from build123d import *

# Parameters (mm, degrees)
BOSS_EXTRUDE1_DEPTH    = 19.05
CONVERT_SOLID1_START   = -19.05
CONVERT_SOLID1_DEPTH   = 38.1
CONVERT_SOLID1_2_DEPTH = 38.1
SKETCH2_W              = 1.8542
SKETCH2_H              = 5.2324
CUT_EXTRUDE1_DEPTH     = 3.175


# Read off the part's stored shape, not the designer's step: SharpBend1
with BuildPart() as part:
    # Sketch1 → Boss-Extrude1 (new, symmetric)
    with BuildSketch(Plane(origin=(0, 0, 0), x_dir=(1, 0, 0), z_dir=(0, 0, -1))):
        Polygon((1.6002, -2.6162), (-6.35, -2.6162), (-6.35, -1.016), (0, -1.016), (0, 1.016), (-6.35, 1.016), (-6.35, 2.6162), (1.6002, 2.6162), align=None)
    extrude(amount=BOSS_EXTRUDE1_DEPTH, both=True)

    # Convert-Solid1 outline → Convert-Solid1 (cut)
    with BuildSketch(Plane.XY.offset(CONVERT_SOLID1_START)):
        with BuildLine():
            Line((1.6002, -2.6162), (1.6002, -0.9906))
            ThreePointArc((1.6002, -0.9906), (1.124072783, -2.140072783), (-0.0254, -2.6162))
            Line((-0.0254, -2.6162), (1.6002, -2.6162))
        make_face()
        with BuildLine():
            ThreePointArc((-0.0254, 2.6162), (1.124072783, 2.140072783), (1.6002, 0.9906))
            Line((1.6002, 0.9906), (1.6002, 2.6162))
            Line((1.6002, 2.6162), (-0.0254, 2.6162))
        make_face()
    extrude(amount=CONVERT_SOLID1_DEPTH, mode=Mode.SUBTRACT)

    # Convert-Solid1 2 outline → Convert-Solid1 2 (add)
    with BuildSketch(Plane.XY.offset(CONVERT_SOLID1_START)):
        with BuildLine():
            Line((0, -1.016), (0, -0.9906))
            ThreePointArc((0, -0.9906), (-0.007439488, -1.008560512), (-0.0254, -1.016))
            Line((-0.0254, -1.016), (0, -1.016))
        make_face()
        with BuildLine():
            ThreePointArc((-0.0254, 1.016), (-0.007439488, 1.008560512), (0, 0.9906))
            Line((0, 0.9906), (0, 1.016))
            Line((0, 1.016), (-0.0254, 1.016))
        make_face()
    extrude(amount=CONVERT_SOLID1_2_DEPTH)

    # Sketch2 → Cut-Extrude1 (cut, symmetric)
    with BuildSketch(Plane.XY):
        with Locations((0.6731, 0)):
            Rectangle(SKETCH2_W, SKETCH2_H)
    extrude(amount=CUT_EXTRUDE1_DEPTH, both=True, mode=Mode.SUBTRACT)


solid = part.part
Here's how the part is built. I have some questions about the finished solid (model axes, mm). A direction names the side the tool comes from. Coordinates: 2 decimals unless noted, no trailing zeros. Order: outer loops, then holes, each group sorted by start corner. A loop starts at its lowest first (then second) coordinate and runs counter-clockwise, first axis right, second up. Notation, with made-up numbers: (-10, 37) - (17, 37) arc R19 cw to (17, 68) - close; hole circle Ø4 at (27, 52.5). An arc over 180 degrees is marked (long way). Use CSV: the item, a comma, the result in double quotes. Start each with the question number.
1. Suppose I cut it at D-D on y = -2.2. List the corners of the cut face in (x, z) for me (3 decimals), then the cut area to 3 significant figures.
2. Suppose I cut it at A-A on y = 0.05. List the corners of the cut face in (x, z) for me (3 decimals), then the cut area to 3 significant figures.
3. Suppose I cut it at B-B on x = -0.75. List the corners of the cut face in (y, z) for me.
4. Please list where these lines run through material, in increasing order: line 1 (Z direction, x = 1.25, y = -0.95) (3 decimals); line 2 (Y direction, x = -3.5, z = -15); line 3 (X direction, y = -1.15, z = 7.5). Write a range as from..to.
5. I'm going to push flat-ended pins straight in: pin 1 (1.6 mm diameter, centred on y = 0, z = 9, fed in from -X); pin 2 (1.3 mm diameter, centred on y = 2, z = -0.5, fed in from +X); pin 3 (2 mm diameter, centred on x = 0.5, z = 8.5, fed in from -Y). Where does each tip first touch, or does it pass through?
6. For faces 5 (the face through (-3, 1.016, 0)), 6 (the face through (-6.35, -2, 0)), 7 (the face through (-0.254, -2, 0)), which set-ups out of +Z, -Z, +X, -X, +Y, -Y let a thin tool reach every point of the face, with its end or its side?
7. If we mould it in two halves opening along Z, with no side actions, what happens to faces 1 (the face through (0, 0, -11)), 2 (the face through (-2.4, 1.2, 19.05)), 3 (the face through (1, 0, 3.175)), 4 (the face through (1, 0, -3.175))? For each: +Z half, -Z half, draft (parallel to the pull), parting line (faces both ways), or undercut.
Output:
1,outline,"(-6.35, -19.05) - (1.061, -19.05) - (1.061, -3.175) - (-0.254, -3.175) - (-0.254, 3.175) - (1.061, 3.175) - (1.061, 19.05) - (-6.35, 19.05) - close"
1,area,"274 mm2"
2,outline,"(0, -19.05) - (1.6, -19.05) - (1.6, -3.175) - (0, -3.175) - close; (0, 3.175) - (1.6, 3.175) - (1.6, 19.05) - (0, 19.05) - close"
2,area,"50.8 mm2"
3,outline,"(-2.62, -19.05) - (-1.02, -19.05) - (-1.02, 19.05) - (-2.62, 19.05) - close; (1.02, -19.05) - (2.62, -19.05) - (2.62, 19.05) - (1.02, 19.05) - close"
4,line 1,"z = -19.05..-3.175, 3.175..19.05"
4,line 2,"y = -2.62..-1.02, 1.02..2.62"
4,line 3,"x = -6.35..1.59"
5,pin 1,"stops at x = 0"
5,pin 2,"stops at x = -0.25"
5,pin 3,"stops at y = -2.62"
6,face 5,"+Z, -Z, -X"
6,face 6,"+Z, -Z, -X, +Y, -Y"
6,face 7,"+X, +Y, -Y"
7,face 1,"draft"
7,face 2,"+Z half"
7,face 3,"undercut"
7,face 4,"undercut"
